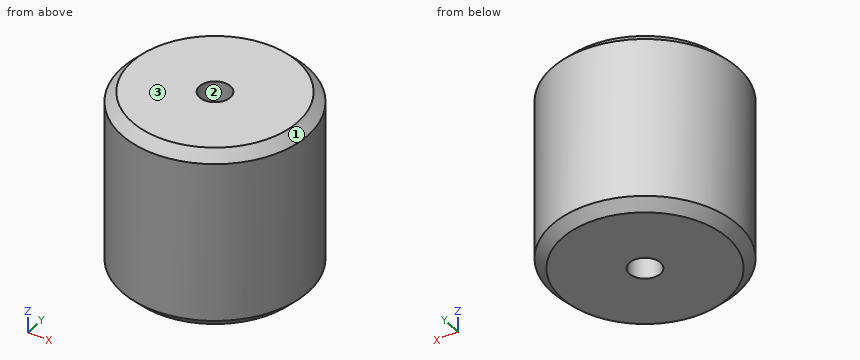
Autodesk Inventor part; units mm, degrees
ref_plane "YZ Plane" through (0, 0, 0) normal (1, 0, 0) x (0, 1, 0)
ref_plane "XZ Plane" through (0, 0, 0) normal (0, 1, 0) x (-1, 0, 0)
ref_plane "XY Plane" through (0, 0, 0) normal (0, 0, 1) x (1, 0, 0)
sketch "Sketch1" plane through (0, 0, 0) normal (0, 0, 1) x (1, 0, 0)
  circle A0 centre (0, 0) radius 9.3
  dimension "d0" = 18.6
extrude "Extrusion1" add sketch "Sketch1" along normal mid plane 18
chamfer "Chamfer1" distance 1 angle 45 2 edges at (-9.3, 0, 9) (-9.3, 0, -9)
sketch "Sketch2" plane through (0, 0, 9) normal (0, 0, 1) x (1, 0, 0)
  circle A0 centre (0, 0) radius 1.55
  dimension "d6" = 3.1
extrude "Extrusion2" cut sketch "Sketch2" against normal blind 18
properties part number "Roller"
Geometry: final body of the model. Coordinates: model frame, mm. Face numbers are marked on the shaded views. Coordinates: 2 decimals unless noted, no trailing zeros. Order: outer loops, then holes, each group sorted by start corner. A loop starts at its lowest first (then second) coordinate and runs counter-clockwise, first axis right, second up. Notation, with made-up numbers: (15.25, 50) -> (73.25, 50) arc R31 cw to (73.25, 75) -> close; hole circle Ø1 at (45.5, 31). An arc over 180 degrees is marked (long way). Answer in a Markdown table with one row per item.
Item 1: Ray query, L1, parallel to Y at x = 0, z = 3.25; L2, parallel to Y at x = 1, z = -6.5. Return the intervals inside material, ascending.
Return value:
| item | result |
|---|---|
| L1 | y = -9.3 to -1.55, 1.55 to 9.3 |
| L2 | y = -9.25 to -1.18, 1.18 to 9.25 |
Item 2: Section C-C on z = 4. Output: boundary loops of the cut face in (x, y).
Return value:
| item | result |
|---|---|
| outline | circle Ø18.6 at (0, 0); hole circle Ø3.1 at (0, 0) |
Item 3: Draft query along X for the marked faces 1, 2 and 3. Return one class per face: released by +X, released by -X, zero draft, split by the parting line, or undercut.
Return value:
| item | result |
|---|---|
| face 1 | split by the parting line |
| face 2 | undercut |
| face 3 | zero draft |
Item 4: Section A-A on y = 0. Output: boundary loops of the cut face in (x, z).
Return value:
| item | result |
|---|---|
| outline | (-9.3, -8) -> (-8.3, -9) -> (-1.55, -9) -> (-1.55, 9) -> (-8.3, 9) -> (-9.3, 8) -> close; (1.55, -9) -> (8.3, -9) -> (9.3, -8) -> (9.3, 8) -> (8.3, 9) -> (1.55, 9) -> close |
